For this review, take the finished solid that the model builds, in its own axes (mm). A direction names the side the tool comes from. Coordinates: 2 decimals unless noted, no trailing zeros. Loops run counter-clockwise (first coordinate to the right, second up) from the corner with the lowest first, then second, coordinate; pieces in that order, holes last. Notation, with made-up numbers: (-27, 46) - (14, 46) arc R32 cw to (14, 78) - close; hole circle Ø6 at (38, 51). An arc over 180 degrees is marked (long way). One line per item, written item: value. Start each with the question number.
1. To check wall thickness, follow line 1 (Y direction, x = 14, z = 45); line 2 (Z direction, x = -55.5, y = -80); line 3 (Y direction, x = -49.5, z = 47). State the ranges of each line that lie inside material, in increasing order. Write a range as from..to.
2. For faces 1 (the face through (1, 1, 2)), 2 (the face through (-75, -160, 43)), 3 (the face through (70, -151, 32)), 4 (the face through (75, -160, 43)), list the 3-axis set-ups (+Z, -Z, +X, -X, +Y, -Y) from which the entire face can be reached by the end or side of a thin tool; tool diameter is ignored.
3. Take a section at D-D, the plane y = 138.5. State the section outline as (x, z) points, and give its area (3 significant figures).
4. Insertion check: pin 1 (1.6 mm diameter, centred on x = -73.5, z = 1, fed in from +Y); pin 2 (2 mm diameter, centred on y = 75.5, z = 1, fed in from -X); pin 3 (1 mm diameter, centred on x = -72, z = 1, fed in from -Y). Each pin has a flat end and moves straight along its axis. Give the tip position at first contact, or say it passes through.
5. Take a section at C-C, the plane y = -92. State the section outline as (x, z) points.
6. Take a section at A-A, the plane x = 24. State the section outline as (y, z) points.
7. The part is to be moulded in two halves that separate along Y. For faces 5 (the face through (1.05, 145.005, 24.548)), 6 (the face through (1.05, -144.43, 25.56)), 7 (the face through (1, -2, 0)), say which applies: released by +Y, released by -Y, zero draft, split by the parting line, or undercut.
8. Take a section at B-B, the plane z = 17. State the section outline as (x, y) points.
```python
from build123d import *

# Parameters (mm, degrees)
F1_DEPTH = 75
F2_W     = 8
F2_H     = 2
F3_DEPTH = 5


with BuildPart() as f1:
    # F0 (on Right) → F1 (new body, symmetric)
    with BuildSketch(Plane.YZ):
        Polygon((-167.3746470185, 49.7928888027), (-125.5934523889, 0), (124.4065476111, 0), (166.1877422407, 49.7928888027), (163.5769276621, 49.7928888027), (123.4739322948, 2), (-124.6608370726, 2), (-164.7638324399, 49.7928888027), align=None)
    extrude(amount=F1_DEPTH, both=True)

    # F2 (on face) → F3 (cut)
    with BuildSketch(Plane.YZ.offset(75)):
        with Locations((-75.5934523889, 1)):
            Rectangle(F2_W, F2_H)
        with Locations((74.4065476111, 1)):
            Rectangle(F2_W, F2_H)
        Polygon((151.7999011608, 35.7575751597), (146.6576002833, 29.6292196148), (148.1896891695, 28.3436443954), (153.331990047, 34.4719999404), align=None)
        Polygon((-149.3765939473, 28.3436443954), (-147.8445050611, 29.6292196148), (-152.9868059385, 35.7575751597), (-154.5188948248, 34.4719999404), align=None)
    extrude(amount=-F3_DEPTH, mode=Mode.SUBTRACT)

    # F4: F1 across plane


with BuildPart() as f1_1:
    add(f1.part)
    add(f1.part.mirror(Plane.YZ), mode=Mode.INTERSECT)


solid = f1_1.part
```
Solutions:
1. line 1: -163.35..-160.74, 159.56..162.17
1. line 2: 0..2
1. line 3: -165.03..-162.42, 161.23..163.84
2. face 1: +Z, +X, -X
2. face 2: +Z, -Z, -X, +Y, -Y
2. face 3: +X
2. face 4: +Z, -Z, +X, +Y, -Y
3. outline: (-75, 16.8) - (75, 16.8) - (75, 19.91) - (-75, 19.91) - close
3. area: 467 mm2
4. pin 1: y = 125.92
4. pin 2: x = -70
4. pin 3: y = -126.85
5. outline: (-75, 0) - (75, 0) - (75, 2) - (-75, 2) - close
6. outline: (-167.37, 49.79) - (-125.59, 0) - (124.41, 0) - (166.19, 49.79) - (163.58, 49.79) - (123.47, 2) - (-124.66, 2) - (-164.76, 49.79) - close
7. face 5: released by +Y
7. face 6: undercut
7. face 7: zero draft
8. outline: (-75, -139.86) - (75, -139.86) - (75, -137.25) - (-75, -137.25) - close; (-75, 136.06) - (75, 136.06) - (75, 138.67) - (-75, 138.67) - close
